Here's how the part is built. I have some questions about the finished solid (model axes, mm). Face numbers are marked on the shaded views. Give positions to 0.01 mm unless a question says otherwise; leave off trailing zeros. Write each loop counter-clockwise with the first axis right and the second up, starting at its lowest first coordinate (ties: lowest second). Pieces come first, ordered by that corner, then holes. Notation, with made-up numbers: (20.5, -35.75) - (76.5, -35.75) arc R18 ccw to (76.5, -0.75) - close; hole circle Ø11 at (44, -40). An arc over 180 degrees is marked (long way). Use a Markdown table: item, result.
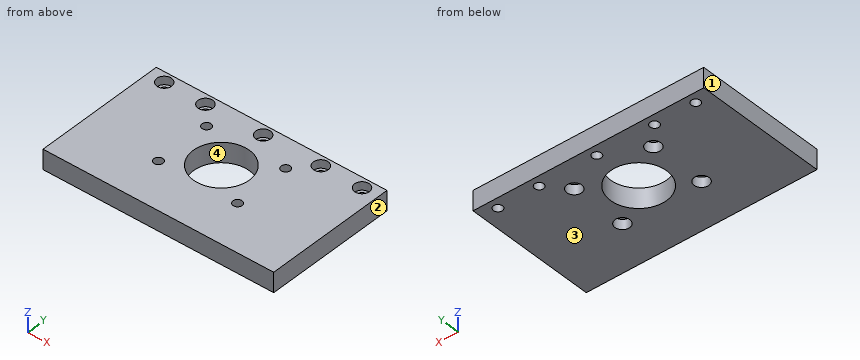
```python
from build123d import *

# Parameters (mm, degrees)
SZKIC1_W                                             = 140
SZKIC1_H                                             = 80
DODANIE_WYCI_GNI_CIE1_DEPTH                          = 12
POG_BIENIE_WALCOWE_POD_M5_WKR_T_DO_CZ_CI_D           = 5.5
POG_BIENIE_WALCOWE_POD_M5_WKR_T_DO_CZ_CI_CBORE_D     = 9
POG_BIENIE_WALCOWE_POD_M5_WKR_T_DO_CZ_CI_CBORE_DEPTH = 5
SZKIC4_R                                             = 17
WYTNIJ_WYCI_GNI_CIE1_DEPTH                           = 156.669521744
POG_BIENIE_WALCOWE_POD_M5_WKR_T_DO_C_2_D             = 5.5
POG_BIENIE_WALCOWE_POD_M5_WKR_T_DO_C_2_CBORE_D       = 9
POG_BIENIE_WALCOWE_POD_M5_WKR_T_DO_C_2_CBORE_DEPTH   = 6


with BuildPart() as part:
    # Szkic1 → Dodanie-wyciągnięcie1 (new body)
    with BuildSketch(Plane.XY):
        with Locations((-70, -27)):
            Rectangle(SZKIC1_W, SZKIC1_H)
    extrude(amount=DODANIE_WYCI_GNI_CIE1_DEPTH)

    # Pog_bienie walcowe pod M5 Wkr_t do cz_ci (through all)
    with Locations(Plane.XY.offset(12)):
        with Locations((-10, 7), (-35, 7), (-105, 7), (-130, 7), (-70, 7)):
            CounterBoreHole(POG_BIENIE_WALCOWE_POD_M5_WKR_T_DO_CZ_CI_D / 2, POG_BIENIE_WALCOWE_POD_M5_WKR_T_DO_CZ_CI_CBORE_D / 2, POG_BIENIE_WALCOWE_POD_M5_WKR_T_DO_CZ_CI_CBORE_DEPTH)

    # Szkic4 → Wytnij-wyciągnięcie1 (cut, through all)
    with BuildSketch(Plane(origin=(0, 0, 0), x_dir=(-1, 0, 0), z_dir=(0, 0, -1))):
        with Locations((70, -22.5)):
            Circle(SZKIC4_R)
    extrude(amount=-WYTNIJ_WYCI_GNI_CIE1_DEPTH, mode=Mode.SUBTRACT)

    # Pog_bienie walcowe pod M5 Wkr_t do c 2 (through all)
    with Locations(Plane(origin=(0, 0, 0), x_dir=(-1, 0, 0), z_dir=(0, 0, -1))):
        with Locations((46, -39), (46, -5)):
            pog_bienie_walcowe_pod_m5_wkr_t_do_c_2 = CounterBoreHole(POG_BIENIE_WALCOWE_POD_M5_WKR_T_DO_C_2_D / 2, POG_BIENIE_WALCOWE_POD_M5_WKR_T_DO_C_2_CBORE_D / 2, POG_BIENIE_WALCOWE_POD_M5_WKR_T_DO_C_2_CBORE_DEPTH)

    # Lustro1: Pog_bienie walcowe pod M5 Wkr_t do c 2 across plane
    add(pog_bienie_walcowe_pod_m5_wkr_t_do_c_2.mirror(Plane.ZY.offset(70)), mode=Mode.SUBTRACT)


solid = part.part
```
Item 1: If we section it at C-C, the plane z = 3: Count the separate pieces of the cut face and the enclosed holes in it, plus the area to 3 significant figures.
Values:
| item | result |
|---|---|
| separate pieces | 1 |
| enclosed holes | 10 |
| area | 9,920 mm2 |
Item 2: Thinking about a two-plate mould opening in X: for the marked faces 1, 2, 3 and 4, which applies, +X half, -X half, draft (parallel to the pull), parting line (faces both ways), or undercut?
Values:
| item | result |
|---|---|
| face 1 | -X half |
| face 2 | +X half |
| face 3 | draft |
| face 4 | undercut |
Item 3: Will these pins go through, and if not, where does the flat tip stop? pin 1 Ø5 at (x, y) = (-70, 7) entering from -Z; pin 2 Ø4.5 at (x, y) = (-47.5, -38) entering from -Z; pin 3 Ø7 at (x, y) = (-130.5, 7) entering from +Z.
Values:
| item | result |
|---|---|
| pin 1 | passes through |
| pin 2 | stops at z = 6 |
| pin 3 | stops at z = 7 |
Item 4: If we section it at B-B, the plane y = -22.5: Write out the boundary of the cut face in (x, z).
Values:
| item | result |
|---|---|
| outline | (-140, 0) - (-87, 0) - (-87, 12) - (-140, 12) - close; (-53, 0) - (0, 0) - (0, 12) - (-53, 12) - close |
Item 5: If we section it at A-A, the plane x = -46: Write out the boundary of the cut face in (y, z).
Values:
| item | result |
|---|---|
| outline | (-67, 0) - (-43.5, 0) - (-43.5, 6) - (-41.75, 6) - (-41.75, 12) - (-67, 12) - close; (-36.25, 6) - (-34.5, 6) - (-34.5, 0) - (-9.5, 0) - (-9.5, 6) - (-7.75, 6) - (-7.75, 12) - (-36.25, 12) - close; (-2.25, 6) - (-0.5, 6) - (-0.5, 0) - (13, 0) - (13, 12) - (-2.25, 12) - close |
Item 6: I need wall thicknesses on line 1 along Y through (x, z) = (-94, 3); line 2 along Y through (x, z) = (-105, 8.6); line 3 along Y through (x, z) = (-10, 3). Which ranges of each line are inside material? Lowest first, please. Write a range as [from, to].
Values:
| item | result |
|---|---|
| line 1 | y = [-67, -43.5], [-34.5, -9.5], [-0.5, 13] |
| line 2 | y = [-67, 2.5], [11.5, 13] |
| line 3 | y = [-67, 4.25], [9.75, 13] |
Item 7: If we section it at D-D, the plane x = -10: Write out the boundary of the cut face in (y, z), plus the area to 4 significant figures.
Values:
| item | result |
|---|---|
| outline | (-67, 0) - (4.25, 0) - (4.25, 7) - (2.5, 7) - (2.5, 12) - (-67, 12) - close; (9.75, 0) - (13, 0) - (13, 12) - (11.5, 12) - (11.5, 7) - (9.75, 7) - close |
| area | 876.5 mm2 |
